Part print with two shaded views. Sizes in mm from the minimum x, y, z corner. A direction names the side the tool comes from. Give positions to 0.01 mm unless a question says otherwise; leave off trailing zeros. Order: outer loops, then holes, each group sorted by start corner. A loop starts at its lowest first (then second) coordinate and runs counter-clockwise, first axis right, second up. Notation, with made-up numbers: (5, 80) -> (58, 80) arc R23 ccw to (58, 91) -> close; hole circle Ø8 at (37, 1.25). An arc over 180 degrees is marked (long way). Answer as CSV lines item,"result".
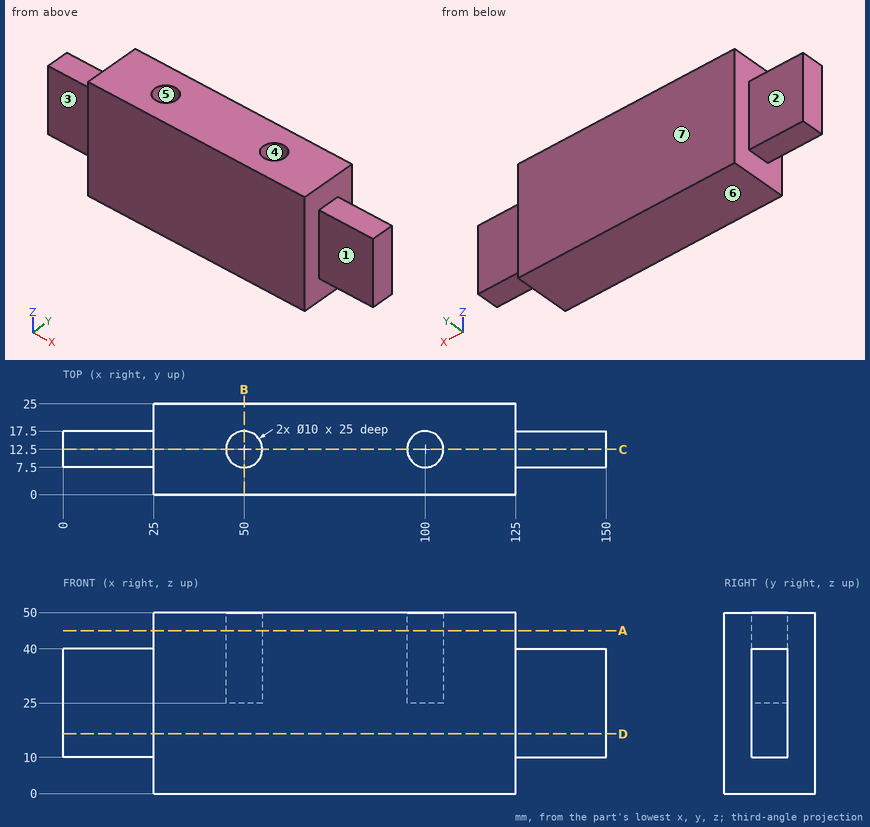
1) Wall check: line 1 along Y through (x, z) = (50, 33.75); line 2 along X through (y, z) = (23.75, 36); line 3 along Z through (x, y) = (130, 12). Give the ranges that are in metal, low to high. Write a range as [from, to].
Data:
line 1,"y = [0, 7.5], [17.5, 25]"
line 2,"x = [25, 125]"
line 3,"z = [10, 40]"
2) Band-saw the part on D-D, the plane z = 16.5. Write the cut outline in (x, y).
Data:
outline,"(0, 7.5) -> (25, 7.5) -> (25, 0) -> (125, 0) -> (125, 7.5) -> (150, 7.5) -> (150, 17.5) -> (125, 17.5) -> (125, 25) -> (25, 25) -> (25, 17.5) -> (0, 17.5) -> close"
3) Pull direction Y, two halves, no side cores. Call the marked faces 4, 5, 6 and 7: pulls with the +Y half, pulls with the -Y half, needs draft (parallel to the pull), parting line crosses it, or undercut.
Data:
face 4,"undercut"
face 5,"undercut"
face 6,"needs draft"
face 7,"pulls with the +Y half"
4) Band-saw the part on B-B, the plane x = 50. Write the cut outline in (y, z).
Data:
outline,"(0, 0) -> (25, 0) -> (25, 50) -> (17.5, 50) -> (17.5, 25) -> (7.5, 25) -> (7.5, 50) -> (0, 50) -> close"
5) Which spindle directions (+Z, -Z, +X, -X, +Y, -Y) get a long thin tool onto all of the face, cutting with end or side? Do the marked faces 1, 2 and 3. Say none if no direction does.
Data:
face 1,"+Z, -Z, +X, -Y"
face 2,"+Z, -Z, -X, +Y"
face 3,"+Z, -Z, -X, -Y"
6) Band-saw the part on C-C, the plane y = 12.5. Write the cut outline in (x, z).
Data:
outline,"(0, 10) -> (25, 10) -> (25, 0) -> (125, 0) -> (125, 10) -> (150, 10) -> (150, 40) -> (125, 40) -> (125, 50) -> (105, 50) -> (105, 25) -> (95, 25) -> (95, 50) -> (55, 50) -> (55, 25) -> (45, 25) -> (45, 50) -> (25, 50) -> (25, 40) -> (0, 40) -> close"
7) Pin check, flat tips, straight feed: P1, Ø4, axis at x = 19, z = 24.5, coming from the -Y side; P2, Ø5, axis at x = 11, y = 15, coming from the +Z side; P3, Ø3, axis at x = 141, y = 13.5, coming from the -Z side. Stop position of each tip, or through.
Data:
P1,"stops at y = 7.5"
P2,"stops at z = 40"
P3,"stops at z = 10"
8) Band-saw the part on A-A, the plane z = 45. Write the cut outline in (x, y), then the cut area to 3 significant figures.
Data:
outline,"(25, 0) -> (125, 0) -> (125, 25) -> (25, 25) -> close; hole circle Ø10 at (50, 12.5); hole circle Ø10 at (100, 12.5)"
area,"2,340 mm2"
